from build123d import *

# Parameters (mm, degrees)
F0_W     = 127
F0_H     = 127
F0_R     = 8.3312
F1_DEPTH = 22.352
F2_R     = 17.526
F3_DEPTH = 25.4
F4_R     = 3.175


with BuildPart() as f1:
    # F0 (on Top) → F1 (new body)
    with BuildSketch(Plane.XY):
        Rectangle(F0_W, F0_H)
        with Locations((-48.387, -48.387)):
            Circle(F0_R, mode=Mode.SUBTRACT)
        with Locations((48.387, -48.387)):
            Circle(F0_R, mode=Mode.SUBTRACT)
        with Locations((-48.387, 48.387)):
            Circle(F0_R, mode=Mode.SUBTRACT)
        with Locations((48.387, 48.387)):
            Circle(F0_R, mode=Mode.SUBTRACT)
    extrude(amount=-F1_DEPTH)

    # F2 (on Right) → F3 (join, symmetric)
    with BuildSketch(Plane.YZ):
        with BuildLine():
            Line((50.8, 0), (33.846452, 62.961747))
            ThreePointArc((33.846452, 62.961747), (0, 88.9), (-33.846452, 62.961747))
            Line((-33.846452, 62.961747), (-50.8, 0))
            Line((-50.8, 0), (50.8, 0))
        make_face()
        with Locations((0, 53.848)):
            Circle(F2_R, mode=Mode.SUBTRACT)
    extrude(amount=F3_DEPTH, both=True)

    # F4
    f4_edges = [f1.edges().sort_by_distance(p)[0] for p in [
        (25.4, 0, 0),
        (0, -50.8, 0),
        (-25.4, 0, 0),
        (0, 50.8, 0),
        (63.5, 0, 0),
        (0, -63.5, 0),
        (-63.5, 0, 0),
        (0, 63.5, 0),
        (25.4, -42.323226, 31.480874),
        (-25.4, -42.323226, 31.480874),
        (63.5, -63.5, -11.176),
        (63.5, 63.5, -11.176),
        (-63.5, -63.5, -11.176),
        (-63.5, 63.5, -11.176),
    ]]
    fillet(f4_edges, radius=F4_R)


solid = f1.part
Geometry: final body of the model. Coordinates: model frame, mm. Give positions to 0.01 mm unless a question says otherwise; leave off trailing zeros. Order: outer loops, then holes, each group sorted by start corner. A loop starts at its lowest first (then second) coordinate and runs counter-clockwise, first axis right, second up. Notation, with made-up numbers: (58, -34) -> (114, -34) arc R21 cw to (114, -11) -> close; hole circle Ø10 at (80, 76.5). An arc over 180 degrees is marked (long way). Write each question's results on one line, items separated by ' | '.
1) Cut plane C-C (x = -11). Output: boundary loops of the cut face in (y, z) (3 decimals).
Geometry says:
outline: (-63.5, -22.352) -> (63.5, -22.352) -> (63.5, -3.175) arc R3.175 ccw to (60.325, 0) -> (53.233, 0) arc R3.175 cw to (50.167, 2.349) -> (33.846, 62.962) arc R35.052 ccw to (-33.846, 62.962) -> (-50.167, 2.349) arc R3.175 cw to (-53.233, 0) -> (-60.325, 0) arc R3.175 ccw to (-63.5, -3.175) -> close; hole circle Ø35.052 at (0, 53.848)
2) First-contact query: pin 1 Ø12 at (x, y) = (8.5, 8) entering from +Z; pin 2 Ø6 at (x, y) = (32, 21) entering from +Z; pin 3 Ø1 at (y, z) = (-20, 36.5) entering from +X. Flat tips, straight axial feed; report the tip coordinate or a pass-through.
Geometry says:
pin 1: stops at z = 88.84 | pin 2: stops at z = 0 | pin 3: stops at x = 25.4
3) Draft query along X for faces 1 (the face through (-62.59, -62.55, -12.9)), 2 (the face through (0.311, -41.893, 33.08)), 3 (the face through (-49.472, -40.127, -11.02)), 4 (the face through (24.445, 41.018, 32.844)). Return one class per face: released by +X, released by -X, zero draft, split by the parting line, or undercut.
Geometry says:
face 1: released by -X | face 2: zero draft | face 3: undercut | face 4: released by +X
4) Cut plane B-B (x = -46). Output: boundary loops of the cut face in (y, z) (3 decimals), and give its area (3 significant figures).
Geometry says:
outline: (-63.5, -22.352) -> (-56.369, -22.352) -> (-56.369, 0) -> (-60.325, 0) arc R3.175 ccw to (-63.5, -3.175) -> close; (-40.405, -22.352) -> (40.405, -22.352) -> (40.405, 0) -> (-40.405, 0) -> close; (56.369, -22.352) -> (63.5, -22.352) -> (63.5, -3.175) arc R3.175 ccw to (60.325, 0) -> (56.369, 0) -> close | area: 2,120 mm²
5) Line query: line 1 along Y through (x, z) = (-41.5, -7.5); line 2 along Y through (x, z) = (-52.5, -8.5); line 3 along Z through (x, y) = (-7, 0). Output: solid intervals per line, ascending.
Geometry says:
line 1: y = -63.5 to -53.08, -43.7 to 43.7, 53.08 to 63.5 | line 2: y = -63.5 to -55.63, -41.14 to 41.14, 55.63 to 63.5 | line 3: z = -22.35 to 36.32, 71.37 to 88.9
6) Cut plane D-D (x = 49). Output: boundary loops of the cut face in (y, z) (3 decimals), and give its area (3 significant figures).
Geometry says:
outline: (-63.5, -22.352) -> (-56.696, -22.352) -> (-56.696, 0) -> (-60.325, 0) arc R3.175 ccw to (-63.5, -3.175) -> close; (-40.078, -22.352) -> (40.078, -22.352) -> (40.078, 0) -> (-40.078, 0) -> close; (56.696, -22.352) -> (63.5, -22.352) -> (63.5, -3.175) arc R3.175 ccw to (60.325, 0) -> (56.696, 0) -> close | area: 2,090 mm²
7) Cut plane A-A (y = 0). Output: boundary loops of the cut face in (x, z) (3 decimals), and give its area (3 significant figures).
Geometry says:
outline: (-63.5, -22.352) -> (63.5, -22.352) -> (63.5, -3.175) arc R3.175 ccw to (60.325, 0) -> (28.575, 0) arc R3.175 cw to (25.4, 3.175) -> (25.4, 36.322) -> (-25.4, 36.322) -> (-25.4, 3.175) arc R3.175 cw to (-28.575, 0) -> (-60.325, 0) arc R3.175 ccw to (-63.5, -3.175) -> close; (-25.4, 71.374) -> (25.4, 71.374) -> (25.4, 85.725) arc R3.175 ccw to (22.225, 88.9) -> (-22.225, 88.9) arc R3.175 ccw to (-25.4, 85.725) -> close | area: 5,570 mm²
